Could you check a few things on this model? Use its own coordinates, in mm. Face numbers are marked on the shaded views. A direction names the side the tool comes from. Give positions to 0.01 mm unless a question says otherwise; leave off trailing zeros. Order: outer loops, then holes, each group sorted by start corner. A loop starts at its lowest first (then second) coordinate and runs counter-clockwise, first axis right, second up.
from build123d import *

# Parameters (mm, degrees)
SKETCH1_W           = 17.135
SKETCH1_H           = 12.5
BASE_DEPTH          = 5
SKETCH2_W           = 17.135
SKETCH2_H           = 15
BOSS_EXTRUDE2_DEPTH = 1.5
BOSS_EXTRUDE3_DEPTH = 17.135
SKETCH4_W           = 11.135
SKETCH4_H           = 15
CUT_EXTRUDE1_DEPTH  = 11
SKETCH5_R           = 1.375
CUT_EXTRUDE2_DEPTH  = 2
SKETCH6_R           = 1.375
CUT_EXTRUDE3_DEPTH  = 5.75
SKETCH7_W           = 17.135
SKETCH7_H           = 12.5
SKETCH7_R           = 1.375
BOSS_EXTRUDE4_DEPTH = 5
SKETCH8_W           = 17.5
SKETCH8_H           = 10
SKETCH8_R           = 1.375
BOSS_EXTRUDE5_DEPTH = 3


with BuildPart() as part:
    # Sketch1 → base (new body)
    with BuildSketch(Plane(origin=(0, 0, 0), x_dir=(1, 0, 0), z_dir=(0, 1, 0))):
        with Locations((8.5675, 6.25)):
            Rectangle(SKETCH1_W, SKETCH1_H)
    extrude(amount=BASE_DEPTH)

    # Sketch2 → Boss-Extrude2 (add)
    with BuildSketch(Plane(origin=(0, 0, -12.5), x_dir=(-1, 0, 0), z_dir=(0, 0, -1))):
        with Locations((-8.5675, -7.5)):
            Rectangle(SKETCH2_W, SKETCH2_H)
    extrude(amount=-BOSS_EXTRUDE2_DEPTH)

    # Sketch3 → Boss-Extrude3 (add)
    with BuildSketch(Plane.ZY):
        Polygon((0, 0), (-11, -15), (-11, 0), align=None)
    extrude(amount=-BOSS_EXTRUDE3_DEPTH)

    # Sketch4 → Cut-Extrude1 (cut)
    with BuildSketch(Plane.XY):
        with Locations((8.5675, -7.5)):
            Rectangle(SKETCH4_W, SKETCH4_H)
    extrude(amount=-CUT_EXTRUDE1_DEPTH, mode=Mode.SUBTRACT)

    # Sketch5 → Cut-Extrude2 (cut)
    with BuildSketch(Plane.XY.offset(-11)):
        with Locations((8.5675, -4)):
            Circle(SKETCH5_R)
        with Locations((8.5675, -11)):
            Circle(SKETCH5_R)
    extrude(amount=-CUT_EXTRUDE2_DEPTH, mode=Mode.SUBTRACT)

    # Sketch6 → Cut-Extrude3 (cut)
    with BuildSketch(Plane(origin=(0, 5, 0), x_dir=(1, 0, 0), z_dir=(0, 1, 0))):
        with Locations((8.5675, 6.25)):
            Circle(SKETCH6_R)
    extrude(amount=-CUT_EXTRUDE3_DEPTH, mode=Mode.SUBTRACT)

    # Sketch7 → Boss-Extrude4 (add)
    with BuildSketch(Plane(origin=(0, 5, 0), x_dir=(1, 0, 0), z_dir=(0, 1, 0))):
        with Locations((8.5675, 6.25)):
            Rectangle(SKETCH7_W, SKETCH7_H)
        with Locations((8.5675, 6.25)):
            Circle(SKETCH7_R, mode=Mode.SUBTRACT)
    extrude(amount=BOSS_EXTRUDE4_DEPTH)

    # Sketch8 → Boss-Extrude5 (add)
    with BuildSketch(Plane(origin=(17.135, 0, 0), x_dir=(0, 0, -1), z_dir=(1, 0, 0))):
        with Locations((-8.75, 5)):
            Rectangle(SKETCH8_W, SKETCH8_H)
        with Locations((-5, 5)):
            Circle(SKETCH8_R, mode=Mode.SUBTRACT)
        with Locations((-12.5, 5)):
            Circle(SKETCH8_R, mode=Mode.SUBTRACT)
    extrude(amount=-BOSS_EXTRUDE5_DEPTH)


solid = part.part
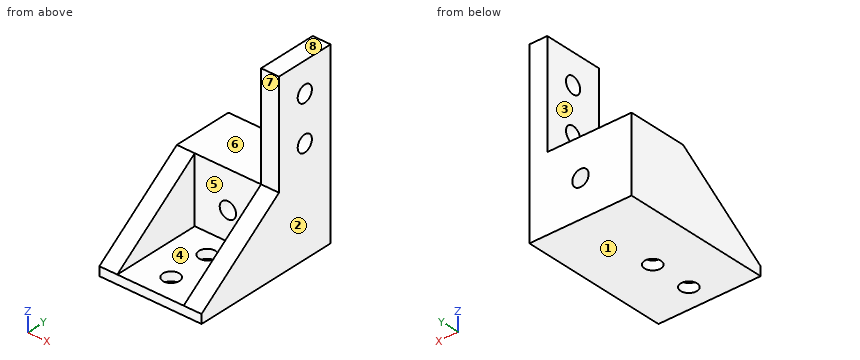
Item 1: For pin 1 (11 mm diameter, centred on y = 5, z = 6.5, fed in from -X) (3 decimals); pin 2 (10 mm diameter, centred on x = 6.5, y = -1, fed in from +Z); pin 3 (5.5 mm diameter, centred on x = 10.5, z = -8, fed in from -Y), each with a flat end and sliding along its axis, tell me the tip position at first contact or that it passes through.
Findings:
pin 1: stops at x = 14.135
pin 2: stops at z = 0
pin 3: stops at y = 0
Item 2: Imagine slicing it at D-D on z = -6.25. List the corners of the cut face in (x, y) for me (1 decimal), then the cut area to 3 significant figures.
Findings:
outline: (0, -8.5) - (3, -8.5) - (3, 0) - (7.2, 0) - (7.2, 10) - (0, 10) - close; (9.9, 0) - (14.1, 0) - (14.1, -8.5) - (17.1, -8.5) - (17.1, 10) - (9.9, 10) - close
area: 195 mm2
Item 3: Imagine slicing it at B-B on x = 12.5. List the corners of the cut face in (y, z) for me.
Findings:
outline: (-15, -12.5) - (10, -12.5) - (10, 0) - (0, 0) - (0, -11) - (-15, -11) - close
Item 4: We'd pull the mould along X, two halves only. Please class the marked faces 1, 2, 3 and 4: +X half, -X half, draft (parallel to the pull), parting line (faces both ways), or undercut.
Findings:
face 1: draft
face 2: +X half
face 3: -X half
face 4: undercut
Item 5: Imagine slicing it at C-C on y = -4. List the corners of the cut face in (x, z) for me (1 decimal).
Findings:
outline: (0, -12.5) - (7.2, -12.5) - (7.2, -11) - (3, -11) - (3, -2.9) - (0, -2.9) - close; (9.9, -12.5) - (17.1, -12.5) - (17.1, -2.9) - (14.1, -2.9) - (14.1, -11) - (9.9, -11) - close
Item 6: Imagine slicing it at A-A on z = 12.5. List the corners of the cut face in (x, y) for me (3 decimals).
Findings:
outline: (14.135, 0) - (17.135, 0) - (17.135, 3.625) - (14.135, 3.625) - close; (14.135, 6.375) - (17.135, 6.375) - (17.135, 10) - (14.135, 10) - close
Item 7: For the marked faces 5, 6, 7 and 8, which set-ups out of +Z, -Z, +X, -X, +Y, -Y let a thin tool reach every point of the face, with its end or its side?
Findings:
face 5: +Z, -Y
face 6: +Z, -X, +Y, -Y
face 7: +Z, +X, -X, -Y
face 8: +Z, +X, -X, +Y, -Y
Item 8: Please list where these lines run through material, in increasing order: line 1 along Y through (x, z) = (16.4, 5) (3 decimals); line 2 along Z through (x, y) = (8.5, 5.25); line 3 along Z through (x, y) = (3.5, -7.25).
Findings:
line 1: y = 0 to 3.625, 6.375 to 10
line 2: z = -12.5 to -7.62, -4.88 to 0
line 3: z = -12.5 to -11
